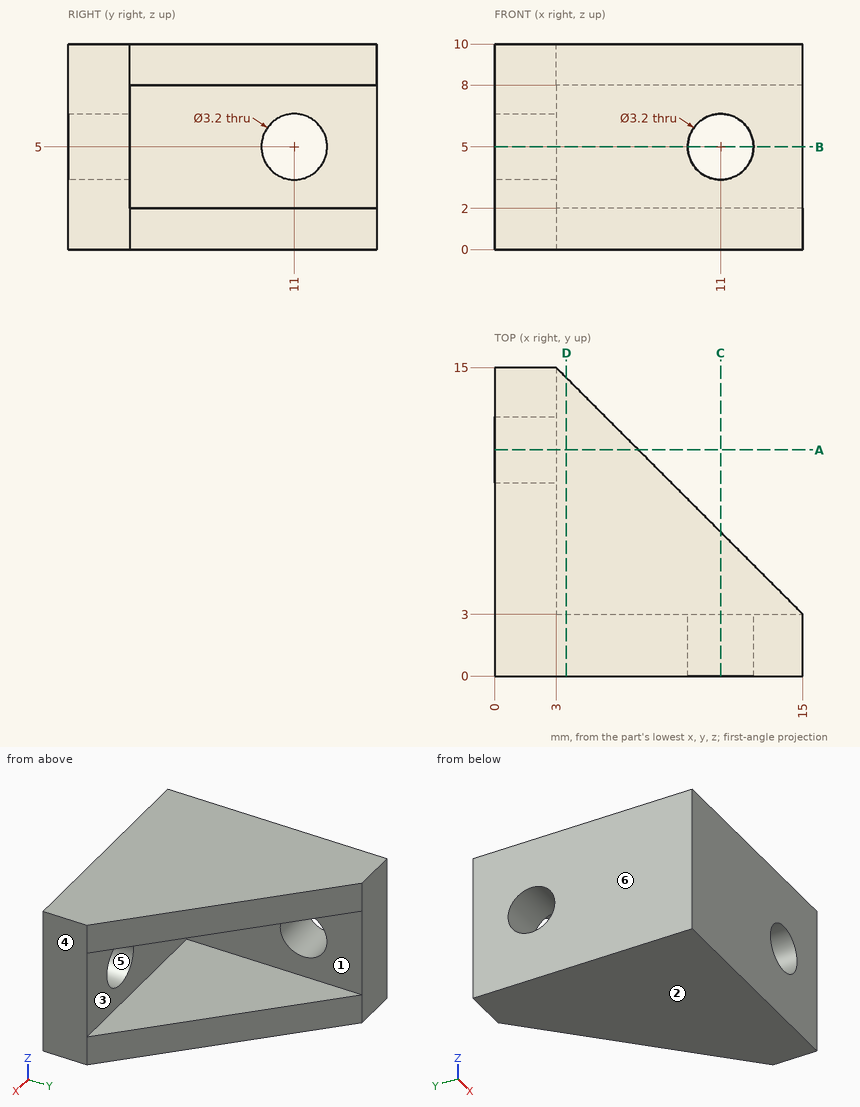
Geometry check sheet. Reference: drawing and pictorial views, mm from the part's lowest x, y, z. A direction names the side the tool comes from. Coordinates: 2 decimals unless noted, no trailing zeros. Order: outer loops, then holes, each group sorted by start corner. A loop starts at its lowest first (then second) coordinate and runs counter-clockwise, first axis right, second up.
Item 1: Material ranges on L1, parallel to Z at x = 7.25, y = 7; L2, parallel to X at y = 1.3, z = 5, recorded low to high.
Filled in:
L1: z = 0 to 2, 8 to 10
L2: x = 0 to 9.4, 12.6 to 15
Item 2: Section check B-B, the plane z = 5. Enter the section's corners in (x, y), then the cut area to 3 significant figures.
Filled in:
outline: (0, 0) - (9.4, 0) - (9.4, 3) - (3, 3) - (3, 9.4) - (0, 9.4) - close; (0, 12.6) - (3, 12.6) - (3, 15) - (0, 15) - close; (12.6, 0) - (15, 0) - (15, 3) - (12.6, 3) - close
area: 61.8 mm2
Item 3: Section check A-A, the plane y = 11. Enter the section's corners in (x, z), then the cut area to 3 significant figures.
Filled in:
outline: (0, 0) - (7, 0) - (7, 2) - (3, 2) - (3, 3.4) - (0, 3.4) - close; (0, 6.6) - (3, 6.6) - (3, 8) - (7, 8) - (7, 10) - (0, 10) - close
area: 36.4 mm2
Item 4: Depth check by flat-ended pin: pin 1 (5 mm diameter, centred on y = 12, z = 1.5, fed in from +X); pin 2 (1.8 mm diameter, centred on x = 10, z = 5, fed in from +Y); pin 3 (3 mm diameter, centred on y = 11, z = 5, fed in from -X); pin 4 (1.8 mm diameter, centred on y = 8, z = 4, fed in from +X). Enter the tip coordinate at first touch or a pass-through.
Filled in:
pin 1: stops at x = 8.5
pin 2: stops at y = 3
pin 3: passes through
pin 4: stops at x = 3
Item 5: Section check D-D, the plane x = 3.5. Enter the section's corners in (y, z), then the cut area to 3 significant figures.
Filled in:
outline: (0, 0) - (14.5, 0) - (14.5, 2) - (3, 2) - (3, 8) - (14.5, 8) - (14.5, 10) - (0, 10) - close
area: 76.0 mm2
Item 6: Access from +Z, -Z, +X, -X, +Y, -Y to the whole of each face (thin tool, end or side, straight path). Record for the marked faces 1 and 2.
Filled in:
face 1: +X, +Y
face 2: -Z, +X, -X, +Y, -Y
Item 7: Release check for a two-part mould opening along X. For the marked faces 3, 4, 5 and 6 record: +X half, -X half, draft (parallel to the pull), parting line (faces both ways), or undercut.
Filled in:
face 3: draft
face 4: +X half
face 5: undercut
face 6: -X half
